Build history of the part. All positions in model axes, mm. A direction names the side the tool comes from. Round coordinates to 2 decimals unless told otherwise and drop trailing zeros. Write each loop counter-clockwise with the first axis right and the second up, starting at its lowest first coordinate (ties: lowest second). Pieces come first, ordered by that corner, then holes. Notation, with made-up numbers: (2.25, -11.5) -> (31.25, -11.5) arc R7 cw to (31.25, -5.5) -> close; hole circle Ø7 at (84, -19). An arc over 180 degrees is marked (long way). One line per question, with ' | ' between items.
Autodesk Inventor part; units mm, degrees
ref_plane "YZ Plane" through (0, 0, 0) normal (1, 0, 0) x (0, 1, 0)
ref_plane "XZ Plane" through (0, 0, 0) normal (0, 1, 0) x (-1, 0, 0)
ref_plane "XY Plane" through (0, 0, 0) normal (0, 0, 1) x (1, 0, 0)
sketch "Sketch1" plane through (0, 0, 0) normal (0, 1, 0) x (-1, 0, 0)
  line L0 (22.4859, 26.2748) -> (64.7859, 26.2748)
  line L1 (64.7859, 26.2748) -> (64.7859, -16.0252)
  line L2 (64.7859, -16.0252) -> (22.4859, -16.0252)
  line L3 (22.4859, -16.0252) -> (22.4859, 26.2748)
  point P0 (0, 0)
  dimension "d0" = 42.3
  dimension "d1" = 42.3
extrude "Extrusion1" add sketch "Sketch1" along normal blind 38
sketch "Sketch2" plane through (0, 38, 0) normal (0, 1, 0) x (1, 0, 0)
  line L0 (-64.7859, -26.2748) -> (-22.4859, -26.2748) construction
  line L1 (-22.4859, -26.2748) -> (-22.4859, 16.0252) construction
  line L2 (-22.4859, 16.0252) -> (-64.7859, 16.0252) construction
  line L3 (-64.7859, 16.0252) -> (-64.7859, -26.2748) construction
  line L4 (-28.1359, -20.6248) -> (-59.1359, -20.6248) construction
  line L5 (-59.1359, -20.6248) -> (-59.1359, 10.3752) construction
  line L6 (-59.1359, 10.3752) -> (-28.1359, 10.3752) construction
  line L7 (-28.1359, 10.3752) -> (-28.1359, -20.6248) construction
  line L8 (-28.1359, -20.6248) -> (-59.1359, 10.3752) construction
  line L9 (-59.1359, -20.6248) -> (-28.1359, 10.3752) construction
  circle A0 centre (-59.1359, -20.6248) radius 1.5
  circle A1 centre (-59.1359, 10.3752) radius 1.5
  circle A2 centre (-28.1359, -20.6248) radius 1.5
  circle A3 centre (-28.1359, 10.3752) radius 1.5
  point P0 (0, 0)
  point P1 (-43.6359, -5.1248)
  dimension "d4" = 31
  dimension "d5" = 31
  dimension "d6" = 3
  dimension "d7" = 3
  dimension "d8" = 3
  dimension "d9" = 3
extrude "Extrusion2" cut sketch "Sketch2" against normal blind 4.5
sketch "Sketch3" plane through (0, 38, 0) normal (0, 1, 0) x (1, 0, 0)
  circle A0 centre (-28.1359, -20.6248) radius 1.5 construction
  circle A1 centre (-59.1359, -20.6248) radius 1.5 construction
  circle A2 centre (-59.1359, 10.3752) radius 1.5 construction
  circle A3 centre (-28.1359, 10.3752) radius 1.5 construction
  line L0 (-64.7859, -26.2748) -> (-22.4859, -26.2748) construction
  line L1 (-22.4859, -26.2748) -> (-22.4859, 16.0252) construction
  line L2 (-22.4859, 16.0252) -> (-64.7859, 16.0252) construction
  line L3 (-64.7859, 16.0252) -> (-64.7859, -26.2748) construction
  circle A4 centre (-43.6359, -5.1248) radius 11
  point P0 (0, 0)
  dimension "d12" = 22
extrude "Extrusion3" add sketch "Sketch3" along normal blind 2
sketch "Sketch4" plane through (-43.6359, 40, 5.1248) normal (0, 1, 0) x (1, 0, 0)
  circle A0 centre (0, 0) radius 11 construction
  circle A1 centre (15.5, -15.5) radius 1.5 construction
  circle A2 centre (-15.5, -15.5) radius 1.5 construction
  circle A3 centre (-15.5, 15.5) radius 1.5 construction
  circle A4 centre (15.5, 15.5) radius 1.5 construction
  line L0 (-21.15, -21.15) -> (21.15, -21.15) construction
  line L1 (21.15, -21.15) -> (21.15, 21.15) construction
  line L2 (21.15, 21.15) -> (-21.15, 21.15) construction
  line L3 (-21.15, 21.15) -> (-21.15, -21.15) construction
  arc A5 (-2.4972, 0.1192) -> (-1.9972, 1.5038) centre (0, 0) ccw
  line L4 (-2.4972, 0.1192) -> (-1.9972, 1.5038)
  point P0 (43.6359, 5.1248)
  dimension "d15" = 5
  dimension "d16" = 0.5
extrude "Extrusion4" add sketch "Sketch4" along normal blind 22
(1) Slice it at B-B (z = 0). Write the cut outline in (x, y), then the cut area to 3 significant figures.
Calculated:
outline: (-64.79, 0) -> (-22.49, 0) -> (-22.49, 38) -> (-33.9, 38) -> (-33.9, 40) -> (-53.37, 40) -> (-53.37, 38) -> (-64.79, 38) -> close | area: 1,650 mm2
(2) Mould opens along Z. For faces 4 (the flat face through (-44, 19, -16.025)), 5 (the flat face through (-59, 33.5, -10)), 6 (the flat face through (-64.786, 19, 5)) say: pulls with the +Z half, pulls with the -Z half, needs draft (parallel to the pull), parting line crosses it, or undercut.
Calculated:
face 4: pulls with the -Z half | face 5: undercut | face 6: needs draft
(3) Slice it at D-D (x = -59.5). Write the cut outline in (y, z), then the cut area to 3 significant figures.
Calculated:
outline: (0, -16.03) -> (38, -16.03) -> (38, -11.83) -> (33.5, -11.83) -> (33.5, -8.92) -> (38, -8.92) -> (38, 19.17) -> (33.5, 19.17) -> (33.5, 22.08) -> (38, 22.08) -> (38, 26.27) -> (0, 26.27) -> close | area: 1,580 mm2
(4) 3-axis set-ups, long thin cutter, end or side, ignore diameter. For faces 1 (the cylindrical face through (-41.253, 50.846, 5.88)), 2 (the flat face through (-22.486, 19, 5)), 3 (the flat face through (-45.887, 50.846, 4.323)): which of +Z, -Z, +X, -X, +Y, -Y reach the whole face in a straight line?
Calculated:
face 1: +Y | face 2: +Z, -Z, +X, +Y, -Y | face 3: -Z, -X, +Y
(5) Drop flat-ended pins along their axis: pin 1 (0.9 mm diameter, centred on x = -29, z = -10, fed in from +Y); pin 2 (3.5 mm diameter, centred on x = -28.14, z = -10.38, fed in from -Y); pin 3 (2.5 mm diameter, centred on x = -59.5, z = -10, fed in from +Y). Give the stop position or say it passes through.
Calculated:
pin 1: y = 33.5 | pin 2: y = 0 | pin 3: y = 38
(6) Slice it at A-A (x = -36). Write the cut outline in (y, z).
Calculated:
outline: (0, -16.03) -> (38, -16.03) -> (38, -2.79) -> (40, -2.79) -> (40, 13.04) -> (38, 13.04) -> (38, 26.27) -> (0, 26.27) -> close
(7) Wall check: line 1 (Y direction, x = -53, z = 16); line 2 (Y direction, x = -37.5, z = 6). Give the ranges that are in metal, low to high. Write a range as from..to.
Calculated:
line 1: 0..38 | line 2: 0..40
(8) Slice it at C-C (y = 48). Write the cut outline in (x, z).
Calculated:
outline: (-46.13, 5.01) -> (-45.63, 3.62) arc R2.5 ccw (long way) to start
